Autodesk Inventor part; units mm, degrees
ref_plane "YZ Plane" through (0, 0, 0) normal (1, 0, 0) x (0, 1, 0)
ref_plane "XZ Plane" through (0, 0, 0) normal (0, 1, 0) x (-1, 0, 0)
ref_plane "XY Plane" through (0, 0, 0) normal (0, 0, 1) x (1, 0, 0)
sketch "Skizze1" plane through (0, 0, 0) normal (0, 0, 1) x (1, 0, 0)
  line L0 (30, 3) -> (30, -3)
  line L1 (30, -3) -> (-3.765, -3)
  line L2 (-3.765, -3) -> (-3.765, 3)
  line L3 (-3.765, 3) -> (30, 3)
  circle A0 centre (0, 0) radius 1.6
  circle A1 centre (0, 0) radius 1.6
  circle A2 centre (27, 0) radius 1.6
  circle A3 centre (27, 0) radius 1.6
  line L4 (21.832, 1.0001) -> (21.832, -3)
  line L5 (21.832, -3) -> (5.832, -3)
  line L6 (5.832, -3) -> (5.832, 1.0001)
  line L7 (5.832, 1.0001) -> (21.832, 1.0001)
  dimension "d0" = 6
extrude "Extrusion1" add sketch "Skizze1" along normal blind 7
sketch "Skizze2" plane through (-3.765, -3, 0) normal (0, -1, 0) x (1, 0, 0)
  line L0 (0, 0) -> (33.765, 0)
  line L1 (0, 0) -> (9.597, 0)
  line L2 (9.597, 0) -> (25.597, 0)
  line L3 (17.597, 0) -> (17.597, -4)
  circle A0 centre (17.597, -4) radius 8
  line L4 (0, 0) -> (0, 2)
  circle A1 centre (17.597, -4) radius 10
  line L5 (0, 2) -> (9.597, 2)
  line L6 (0, 0) -> (0, 7)
  line L7 (33.765, 0) -> (33.765, 2)
  line L8 (33.765, 0) -> (33.765, 7)
  line L9 (33.765, 2) -> (25.597, 2)
  line L10 (33.765, 7) -> (0, 7)
  line L11 (0, 7) -> (33.765, 7)
  line L12 (33.765, 7) -> (33.765, 0)
  line L13 (33.765, 0) -> (0, 0)
  line L14 (0, 0) -> (0, 7)
  point P0 (3.765, 0)
  point P1 (24.5252, 0)
  point P2 (10.6688, 0)
  point P3 (17.597, 7)
  point P4 (8.4318, 0)
  point P5 (26.7622, 0)
  dimension "d3" = 9.597
  dimension "d4" = 16
  dimension "d5" = 4
  dimension "d6" = 16
  dimension "d7" = 2
  dimension "d8" = 2
  dimension "d9" = 2
extrude "Extrusion2" cut sketch "Skizze2" against normal blind 7 contours L6 L10 L8 L9 A1 L5 | A0 L0 picked at (13.3479, 0.4966)
fillet "Rundung1" radius 2 4 edges at (5.832, 0, 2) (6.9038, 0, 0) (20.7602, 0, 0) (21.832, 0, 2)
fillet "Rundung2" radius 1 4 edges at (-3.765, -3, 1) (30, -3, 1) (30, 3, 1) (-3.765, 3, 1)
sketch "Skizze3" plane through (13.832, -3, -4) normal (0, -1, 0) x (1, 0, 0)
  line L0 (-13.832, 4) -> (-6.832, 4)
  line L1 (-15.432, 3) -> (-12.232, 3)
  line L2 (-6.832, 4) -> (-6.832, 13)
  line L3 (-6.832, 13) -> (6.168, 13)
  line L4 (6.168, 13) -> (6.168, 10)
  line L5 (6.168, 10) -> (5.168, 10)
  line L6 (5.168, 10) -> (5.168, 12)
  line L7 (5.168, 12) -> (-4.832, 12)
  line L8 (-4.832, 12) -> (-4.832, 8.7551)
  arc A0 (7.4536, 6.6667) -> (-7.4536, 6.6667) centre (0, 0) ccw
  arc A1 (7.4536, 6.6667) -> (-7.4536, 6.6667) centre (0, 0) ccw
  point P0 (-13.832, 4)
  point P1 (-12.232, 3)
  point P2 (-6.832, 7.3023)
  point P3 (9.1652, 4)
  point P4 (-9.1652, 4)
  dimension "d14" = 7
  dimension "d15" = 9
  dimension "d16" = 13
  dimension "d17" = 3
  dimension "d18" = 1
  dimension "d19" = 2
  dimension "d20" = 10
extrude "Extrusion3" add sketch "Skizze3" against normal up to surface (6 mm away)
fillet "Rundung3" radius 1 7 edges at (20, 0, 6) (20, 0, 9) (7, 0, 9) (19, 0, 8) (9, 0, 8) (9, 0, 4.7551) (7, 0, 3.3023)
fillet "Rundung4" radius 0.2 2 edges at (19.0001, 0, 6) (19, 0, 6)
properties part number "DribblerMotorKlemme"
Model file for the job. Use its own axes, mm. A direction names the side the tool comes from. Coordinates: 2 decimals unless noted, no trailing zeros. Order: outer loops, then holes, each group sorted by start corner. A loop starts at its lowest first (then second) coordinate and runs counter-clockwise, first axis right, second up. Notation, with made-up numbers: (-29, 69) -> (21, 69) arc R25 cw to (21, 92) -> close; hole circle Ø8 at (3.5, -19). An arc over 180 degrees is marked (long way). Answer as a JSON object with one key per item and string values. Group by question number.
1) Cut at C-C, the plane x = 26.5. Write the cut outline in (y, z).
2) Cut at B-B, the plane y = 0.35. Count the separate pieces of the cut face and the enclosed holes in it, then the cut area to 3 significant figures.
3) Pull direction X, two halves, no side cores. Call faces 1 (the face through (14, 0, 8)), 2 (the face through (21.97, 0.04, 2.17)), 3 (the face through (-3.464, 2.715, 1.014)): +X half, -X half, draft (parallel to the pull), parting line (faces both ways), or undercut.
4) Cut at A-A, the plane x = 0. Write the cut outline in (y, z).
5) Flat gauge pins, fed straight in: pin 1 (3 mm diameter, centred on x = 25, y = -0.5, fed in from +Z); pin 2 (0.8 mm diameter, centred on y = 0.5, z = 7, fed in from +X); pin 3 (2 mm diameter, centred on y = 0.5, z = 6, fed in from -X). Where does each tip first touch, or does it go through?
6) Cut at D-D, the plane x = 8.5. Write the cut outline in (y, z), then the cut area to 3 significant figures.
7) Which spindle directions (+Z, -Z, +X, -X, +Y, -Y) get a long thin tool onto all of the face, cutting with end or side? Do faces 4 (the face through (9.418, -0.042, 5.498)), 5 (the face through (6.7, 0, 0.2)), 6 (the face through (7, 0, 6)), 7 (the face through (19.8, 0, 6.4)), 8 (the face through (25.82, -1.08, 0.99)). Say none if no direction does.
8) Drill centre lines: L1, parallel to Y at x = 27, z = 0.7; L2, parallel to X at y = 0, z = 0.95 (3 decimals); L3, parallel to X at y = -1.4, z = 7. Where is each one in solid material? Low to high.
Check values:
{
 "1": {"outline": "(-3, 0) -> (-1.52, 0) -> (-1.52, 2) -> (-3, 2) -> close; (1.52, 0) -> (3, 0) -> (3, 2) -> (1.52, 2) -> close"},
 "2": {"separate pieces": "3", "enclosed holes": "0", "area": "83.5 mm²"},
 "3": {"face 1": "undercut", "face 2": "+X half", "face 3": "-X half"},
 "4": {"outline": "(-3, 0) -> (-1.6, 0) -> (-1.6, 2) -> (-3, 2) -> close; (1.6, 0) -> (3, 0) -> (3, 2) -> (1.6, 2) -> close"},
 "5": {"pin 1": "stops at z = 2", "pin 2": "stops at x = 20", "pin 3": "stops at x = 7"},
 "6": {"outline": "(-3, 1.96) -> (3, 1.96) -> (3, 9) -> (-3, 9) -> close", "area": "42.2 mm²"},
 "7": {"face 4": "+Y, -Y", "face 5": "-Z, +Y, -Y", "face 6": "+Z, -X, +Y, -Y", "face 7": "+X, +Y, -Y", "face 8": "+Z, -Z"},
 "8": {"L1": "y = -3 to -1.6, 1.6 to 3", "L2": "x = -3.765 to -1.6, 1.6 to 7.547, 20.117 to 25.4, 28.6 to 30", "L3": "x = 7 to 9, 19 to 20"}
}
